from build123d import *

# Parameters (mm, degrees)
SKETCH006_R  = 3.2
PAD004_DEPTH = 4.9
SKETCH007_W  = 10
SKETCH007_H  = 10
PAD005_DEPTH = 5.2
SKETCH010_R  = 3.2
PAD006_DEPTH = 4.9
FILLET005_R  = 5


with BuildPart() as part:
    # Sketch006 → Pad004 (new body)
    with BuildSketch(Plane.XY):
        with BuildLine():
            Line((-18, 20), (-13, 20))
            Line((-13, 20), (-13, 0))
            Line((-13, 0), (13, 0))
            Line((13, 0), (13, 20))
            Line((13, 20), (18, 20))
            ThreePointArc((23, 15), (21.535534, 18.535534), (18, 20))
            Line((23, 15), (23, -10))
            Line((23, -10), (-23, -10))
            Line((-23, -10), (-23, 15))
            ThreePointArc((-18, 20), (-21.535534, 18.535534), (-23, 15))
        make_face()
        with Locations((-18, 15)):
            Circle(SKETCH006_R, mode=Mode.SUBTRACT)
        with Locations((18, 15)):
            Circle(SKETCH006_R, mode=Mode.SUBTRACT)
    extrude(amount=PAD004_DEPTH)

    # Sketch007 → Pad005 (new body)
    with BuildSketch(Plane.XY.offset(4.9)):
        with Locations((-18, -5)):
            Rectangle(SKETCH007_W, SKETCH007_H)
        with Locations((18, -5)):
            Rectangle(SKETCH007_W, SKETCH007_H)
    extrude(amount=PAD005_DEPTH)

    # Sketch010 → Pad006 (new body)
    with BuildSketch(Plane.XY.offset(10.1)):
        with BuildLine():
            Line((-18, 20), (-13, 20))
            Line((-13, 20), (-13, 0))
            Line((-13, 0), (13, 0))
            Line((13, 0), (13, 20))
            Line((13, 20), (18, 20))
            ThreePointArc((23, 15), (21.535534, 18.535534), (18, 20))
            Line((23, 15), (23, -10))
            Line((23, -10), (-23, -10))
            Line((-23, -10), (-23, 15))
            ThreePointArc((-18, 20), (-21.535534, 18.535534), (-23, 15))
        make_face()
        with Locations((-18, 15)):
            Circle(SKETCH010_R, mode=Mode.SUBTRACT)
        with Locations((18, 15)):
            Circle(SKETCH010_R, mode=Mode.SUBTRACT)
    extrude(amount=PAD006_DEPTH)

    # Fillet005
    fillet005_edges = [part.edges().sort_by_distance(p)[0] for p in [
        (23, -10, 12.55),
        (23, -10, 7.5),
        (23, -10, 2.45),
        (-23, -10, 2.45),
        (-23, -10, 7.5),
        (-23, -10, 12.55),
    ]]
    fillet(fillet005_edges, radius=FILLET005_R)


solid = part.part
Check sheet for the modelled part. Datum: model origin and axes. Units: mm. A direction names the side the tool comes from. Round coordinates to 2 decimals unless told otherwise and drop trailing zeros. Write each loop counter-clockwise with the first axis right and the second up, starting at its lowest first coordinate (ties: lowest second). Pieces come first, ordered by that corner, then holes. Notation, with made-up numbers: (-16.5, 40.5) - (34.5, 40.5) arc R25 cw to (34.5, 60.5) - close; hole circle Ø11 at (41.25, -19.75). An arc over 180 degrees is marked (long way). Return JSON: item names as keys, results as strings.
Q1. Cross-section at C-C (y = -4.5). Record the boundary of the cut face in (x, z).
Returned:
{"outline": "(-23, 0) - (23, 0) - (23, 15) - (-23, 15) - close; hole (-13, 4.9) - (13, 4.9) - (13, 10.1) - (-13, 10.1) - close"}
Q2. Cross-section at A-A (x = -9). Record the boundary of the cut face in (y, z), then the cut area to 3 significant figures.
Returned:
{"outline": "(-10, 0) - (0, 0) - (0, 4.9) - (-10, 4.9) - close; (-10, 10.1) - (0, 10.1) - (0, 15) - (-10, 15) - close", "area": "98.0 mm²"}
Q3. Depth check by flat-ended pin: P1, Ø2, axis at x = 15.5, y = 3.5, coming from the -Z side; P2, Ø1.5, axis at x = 4, z = 3.5, coming from the +Y side. Enter the tip coordinate at first touch or a pass-through.
Returned:
{"P1": "stops at z = 0", "P2": "stops at y = 0"}
Q4. Cross-section at B-B (z = 2). Record the boundary of the cut face in (x, y), then the cut area to 3 significant figures.
Returned:
{"outline": "(-23, -5) arc R5 ccw to (-18, -10) - (18, -10) arc R5 ccw to (23, -5) - (23, 15) arc R5 ccw to (18, 20) - (13, 20) - (13, 0) - (-13, 0) - (-13, 20) - (-18, 20) arc R5 ccw to (-23, 15) - close; hole circle Ø6.4 at (-18, 15); hole circle Ø6.4 at (18, 15)", "area": "774 mm²"}
Q5. Scan lines: L1, parallel to Z at x = 13.5, y = 6; L2, parallel to Y at x = 18, z = 11.5; L3, parallel to X at y = 3, z = 3.5. Record each from-to range of solid material in increasing order. Write a range as from..to.
Returned:
{"L1": "z = 0..4.9, 10.1..15", "L2": "y = -10..11.8, 18.2..20", "L3": "x = -23..-13, 13..23"}
Q6. Draft check along Y on faces 1 (the flat face through (0, -1, 0)), 2 (the cylindrical face through (-18.694, 11.876, 12.516)), 3 (the cylindrical face through (-21, -9, 8)). Enter one of: released by +Y, released by -Y, zero draft, split by the parting line, or undercut.
Returned:
{"face 1": "zero draft", "face 2": "undercut", "face 3": "released by -Y"}
Q7. Cross-section at D-D (z = 6.75). Record the boundary of the cut face in (x, y).
Returned:
{"outline": "(-23, -5) arc R5 ccw to (-18, -10) - (-13, -10) - (-13, 0) - (-23, 0) - close; (13, -10) - (18, -10) arc R5 ccw to (23, -5) - (23, 0) - (13, 0) - close"}
Q8. Access from +Z, -Z, +X, -X, +Y, -Y to the whole of each face (thin tool, end or side, straight path). Record for faces 4 (the flat face through (0, 0, 13)), 5 (the flat face through (0, -5, 10.1)), 6 (the flat face through (15, 20, 2)), 7 (the flat face through (-18, 8, 4.9)).
Returned:
{"face 4": "+Z, -Z, +Y", "face 5": "+Y, -Y", "face 6": "+Z, -Z, +X, -X, +Y", "face 7": "+X, -X, +Y"}
